from build123d import *

# Parameters (mm, degrees)
F1_DEPTH = 1237.5


with BuildPart() as f1:
    # F0 (on Front) → F1 (new body, symmetric)
    with BuildSketch(Plane.XZ):
        with BuildLine():
            ThreePointArc((25, 10), (24.267766953, 11.767766953), (22.5, 12.5))
            Line((22.5, 12.5), (-22.5, 12.5))
            ThreePointArc((-22.5, 12.5), (-24.267766953, 11.767766953), (-25, 10))
            Line((-25, 10), (-25, -10))
            ThreePointArc((-25, -10), (-24.267766953, -11.767766953), (-22.5, -12.5))
            Line((-22.5, -12.5), (22.5, -12.5))
            ThreePointArc((22.5, -12.5), (24.267766953, -11.767766953), (25, -10))
            Line((25, -10), (25, 10))
        make_face()
        with BuildLine():
            ThreePointArc((22.5, 11), (23.2071067812, 10.7071067812), (23.5, 10))
            Line((23.5, 10), (23.5, -10))
            ThreePointArc((23.5, -10), (23.2071067812, -10.7071067812), (22.5, -11))
            Line((22.5, -11), (-22.5, -11))
            ThreePointArc((-22.5, -11), (-23.2071067812, -10.7071067812), (-23.5, -10))
            Line((-23.5, -10), (-23.5, 10))
            ThreePointArc((-23.5, 10), (-23.2071067812, 10.7071067812), (-22.5, 11))
            Line((-22.5, 11), (22.5, 11))
        make_face(mode=Mode.SUBTRACT)
    extrude(amount=F1_DEPTH, both=True)


solid = f1.part
Source: CAD feature listing. Evaluate the final solid. Frame: model axes, mm. Give positions to 0.01 mm unless a question says otherwise; leave off trailing zeros. Write each loop counter-clockwise with the first axis right and the second up, starting at its lowest first coordinate (ties: lowest second). Pieces come first, ordered by that corner, then holes. Notation, with made-up numbers: M 41.5,59 L 97.5,59 A9 cw 97.5,64 Z; hole C 49.5,86 d3. An arc over 180 degrees is marked long. Return JSON: item names as keys, results as strings. Group by question number.
1) Material intervals for line 1 along X through (y, z) = (-1082.5, 4.5); line 2 along Z through (x, y) = (-13, 577.5); line 3 along X through (y, z) = (176, -10.5), sorted ascending. Write a range as [from, to].
2) Cut plane B-B, the plane x = -7. Output: boundary loops of the cut face in (y, z), plus the area to 4 significant figures.
3) Pull-direction query (Z, two-part tool) for faces 1 (the face through (0, -17, 12.5)), 2 (the face through (0, -17, -12.5)), 3 (the face through (0, -17, 11)); classes: pulls with the +Z half, pulls with the -Z half, needs draft (parallel to the pull), parting line crosses it, or undercut.
4) Cut plane C-C, the plane z = 5.5. Output: boundary loops of the cut face in (x, y), plus the area to 4 significant figures.
5) Cut plane A-A, the plane y = -750. Output: boundary loops of the cut face in (x, z), plus the area to 3 significant figures.
Recorded:
{
 "1": {"line 1": "x = [-25, -23.5], [23.5, 25]", "line 2": "z = [-12.5, -11], [11, 12.5]", "line 3": "x = [-24.95, -23.37], [23.37, 24.95]"},
 "2": {"outline": "M -1237.5,-12.5 L 1237.5,-12.5 L 1237.5,-11 L -1237.5,-11 Z; M -1237.5,11 L 1237.5,11 L 1237.5,12.5 L -1237.5,12.5 Z", "area": "7,425 mm²"},
 "3": {"face 1": "pulls with the +Z half", "face 2": "pulls with the -Z half", "face 3": "undercut"},
 "4": {"outline": "M -25,-1237.5 L -23.5,-1237.5 L -23.5,1237.5 L -25,1237.5 Z; M 23.5,-1237.5 L 25,-1237.5 L 25,1237.5 L 23.5,1237.5 Z", "area": "7,425 mm²"},
 "5": {"outline": "M -25,-10 A2.5 ccw -22.5,-12.5 L 22.5,-12.5 A2.5 ccw 25,-10 L 25,10 A2.5 ccw 22.5,12.5 L -22.5,12.5 A2.5 ccw -25,10 Z; hole M -23.5,-10 A1 ccw -22.5,-11 L 22.5,-11 A1 ccw 23.5,-10 L 23.5,10 A1 ccw 22.5,11 L -22.5,11 A1 ccw -23.5,10 Z", "area": "211 mm²"}
}
